Geometry check sheet. Reference: the model listing, model coordinates, mm. A direction names the side the tool comes from. Coordinates: 2 decimals unless noted, no trailing zeros. Loops run counter-clockwise (first coordinate to the right, second up) from the corner with the lowest first, then second, coordinate; pieces in that order, holes last. Notation, with made-up numbers: (-16, 38) -> (7, 38) arc R21 ccw to (7, 62) -> close; hole circle Ø2 at (33.25, 49.25). An arc over 180 degrees is marked (long way). Answer as a JSON object with one key per item and string values.
from build123d import *

# Parameters (mm, degrees)
F1_DEPTH = 50
F2_R     = 4
F3_DEPTH = 10


with BuildPart() as f1:
    # F0 (on Front) → F1 (new body)
    with BuildSketch(Plane.XZ):
        Polygon((11.096148, 22.337567), (-11.187021, 22.337567), (-11.187021, 9.424148), (0.017039, 9.424148), (11.096148, 9.424148), align=None)
    extrude(amount=F1_DEPTH)

    # F2 (on face) → F3 (cut)
    with BuildSketch(Plane.YZ.offset(11.096148)):
        with Locations((-23, 15.585567)):
            Circle(F2_R)
    extrude(amount=-F3_DEPTH, mode=Mode.SUBTRACT)


solid = f1.part
1. Section check A-A, the plane y = -26.5. Record the boundary of the cut face in (x, z), then the cut area to 3 significant figures.
Evaluation:
{"outline": "(-11.19, 9.42) -> (11.1, 9.42) -> (11.1, 13.65) -> (1.1, 13.65) -> (1.1, 17.52) -> (11.1, 17.52) -> (11.1, 22.34) -> (-11.19, 22.34) -> close", "area": "249 mm^2"}
2. Thickness scan on probe 1 along Y at (x, z) = (7.25, 15.5); probe 2 along Z at (x, y) = (7.5, -23); probe 3 along X at (y, z) = (-24.5, 12.25). Record the ranges inside material, lowest first. Write a range as from..to.
Evaluation:
{"probe 1": "y = -50..-27, -19..0", "probe 2": "z = 9.42..11.59, 19.59..22.34", "probe 3": "x = -11.19..1.1"}
3. Section check B-B, the plane z = 17.75. Record the boundary of the cut face in (x, y).
Evaluation:
{"outline": "(-11.19, -50) -> (11.1, -50) -> (11.1, -26.36) -> (1.1, -26.36) -> (1.1, -19.64) -> (11.1, -19.64) -> (11.1, 0) -> (-11.19, 0) -> close"}
4. Depth check by flat-ended pin: P1, Ø6.5, axis at y = -23, z = 15.59, coming from the +X side. Enter the tip coordinate at first touch or a pass-through.
Evaluation:
{"P1": "stops at x = 1.1"}
5. Tool access check on faces 4 (the face through (1.096, -23, 16)), 5 (the face through (0, -50, 16)). Record the directions out of +Z, -Z, +X, -X, +Y, -Y that give a thin tool (end or side, any length) a straight path to the whole face; none if there is none.
Evaluation:
{"face 4": "+X", "face 5": "+Z, -Z, +X, -X, -Y"}
6. Mould release check, pull along Z, two halves, no side actions. Record for faces 1 (the face through (0, -25, 22.338)), 2 (the face through (6.166, -26.174, 13.152)), 3 (the face through (0, 0, 16)): released by +Z, released by -Z, zero draft, split by the parting line, or undercut.
Evaluation:
{"face 1": "released by +Z", "face 2": "undercut", "face 3": "zero draft"}
